```python
from build123d import *

# Parameters (mm, degrees)
F1_DEPTH = 95.25
F2_R     = 10.16
F2_W     = 39.37
F2_H     = 19.05
F3_DEPTH = 25.4


with BuildPart() as f1:
    # F0 (on Right) → F1 (new body)
    with BuildSketch(Plane.YZ):
        with BuildLine():
            ThreePointArc((42.311873, 41.937777), (13.84255, 32.215467), (-8.645249, 12.232359))
            Line((-8.645249, 12.232359), (-53.689915, -47.56531))
            Line((-53.689915, -47.56531), (-49.879915, -47.56531))
            Line((-49.879915, -47.56531), (-4.835249, 12.232359))
            ThreePointArc((-4.835249, 12.232359), (15.95876, 30.240728), (42.311873, 38.127777))
            Line((42.311873, 38.127777), (42.311873, 41.937777))
        make_face()
    extrude(amount=F1_DEPTH)

    # F2 (on face) → F3 (cut)
    with BuildSketch(Plane(origin=(0, -11.394199, 8.583075), x_dir=(1, 0, 0), z_dir=(0, -0.798739, 0.601678))):
        with Locations((15.24, -49.976293)):
            Circle(F2_R)
        with Locations((47.625, -51.881293)):
            Rectangle(F2_W, F2_H)
        with Locations((80.01, -49.976293)):
            Circle(F2_R)
    extrude(amount=-F3_DEPTH, mode=Mode.SUBTRACT)


solid = f1.part
```
Here's how the part is built. I have some questions about the finished solid (model axes, mm). Give positions to 0.01 mm unless a question says otherwise; leave off trailing zeros. Loops run counter-clockwise (first coordinate to the right, second up) from the corner with the lowest first, then second, coordinate; pieces in that order, holes last. Notation, with made-up numbers: M 29.5,38 L 77.5,38 A24 cw 77.5,64 Z; hole C -24,74 d3. An arc over 180 degrees is marked long. Use one line per item in the form item = value. Start each with the question number.
Q1. I need wall thicknesses on line 1 along Y through (x, z) = (43.5, 11.5); line 2 along Z through (x, y) = (63.5, -4); line 3 along Y through (x, z) = (62.5, 10.5). Which ranges of each line are inside material? Lowest first, please.
Q2. Thinking about a two-plate mould opening in X: for faces 1 (the flat face through (95.25, -13, 4)), 2 (the flat face through (67.31, -41, -34)), 3 (the flat face through (0, -13, 4)), 4 (the cylindrical face through (46.96, 14.21, 32.43)), which applies, +X half, -X half, draft (parallel to the pull), parting line (faces both ways), or undercut?
Q3. If we section it at D-D (z = 32): Write out the boundary of the cut face in (x, y), then the cut area to 3 significant figures.
Q4. If we section it at A-A (x = 49): Write out the boundary of the cut face in (y, z).
Q5. If we section it at C-C (x = 87): Write out the boundary of the cut face in (y, z), then the cut area to 3 significant figures.
Q6. If we section it at B-B (y = -44.5): State how many separate pieces and enclosed holes the cut face has, then the cut area to 3 significant figures.
Q7. Will these pins go through, and if not, where does the flat tip stop? pin 1 Ø6 at (x, z) = (20, 31) entering from -Y; pin 2 Ø1 at (x, y) = (15, -20) entering from +Z; pin 3 Ø1 at (x, y) = (30, -11.5) entering from +Z; pin 4 Ø4 at (y, z) = (-44, -31) entering from +X.
Taken from the geometry:
q1.line_1 = -9.2 to -5.39
q1.line_2 = 13.32 to 17.82
q1.line_3 = -9.95 to -6.14
q2.face_1 = +X half
q2.face_2 = undercut
q2.face_3 = -X half
q2.face_4 = draft
q3.outline = M 0,13.48 L 95.25,13.48 L 95.25,19.4 L 0,19.4 Z
q3.area = 564 mm^2
q4.outline = M -53.69,-47.57 L -49.88,-47.57 L -45.91,-42.3 L -48.34,-40.46 Z; M -36.88,-25.25 L -34.45,-27.08 L -4.84,12.23 A65.53 cw 42.31,38.13 L 42.31,41.94 A76.2 ccw -8.65,12.23 Z
q5.outline = M -53.69,-47.57 L -49.88,-47.57 L -43.47,-39.06 L -45.9,-37.22 Z; M -37.03,-25.45 L -34.6,-27.28 L -4.84,12.23 A65.53 cw 42.31,38.13 L 42.31,41.94 A76.2 ccw -8.65,12.23 Z
q5.area = 356 mm^2
q6.separate_pieces = 4
q6.enclosed_holes = 0
q6.area = 139 mm^2
q7.pin_1 = 7.39
q7.pin_2 = -2.18
q7.pin_3 = 9.11
q7.pin_4 = through
